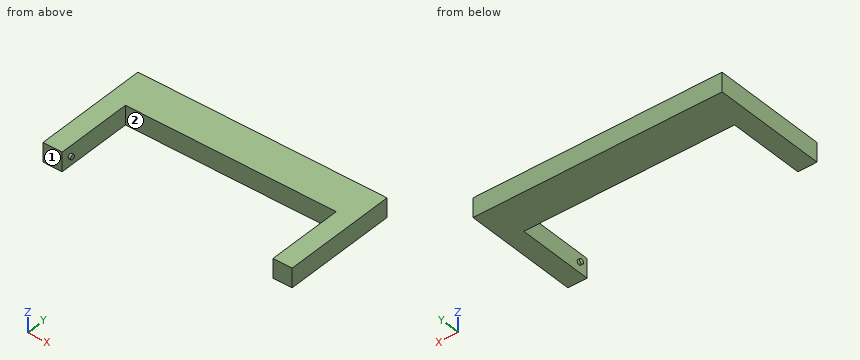
```python
from build123d import *

# Parameters (mm, degrees)
F0_W     = 279.4
F0_H     = 50.8
F1_DEPTH = 25.4
F2_R     = 3.175
F3_DEPTH = 3.175


with BuildPart() as f1:
    # F0 (on Top) → F1 (new body)
    with BuildSketch(Plane.XY):
        with Locations((0, 52.668456)):
            Rectangle(F0_W, F0_H)
        Polygon((-139.7, -74.331544), (-139.7, 27.268456), (-139.7, 78.068456), (-165.1, 78.068456), (-165.1, -74.331544), align=None)
        Polygon((139.7, 78.068456), (139.7, 27.268456), (139.7, -74.331544), (165.1, -74.331544), (165.1, 78.068456), align=None)
    extrude(amount=F1_DEPTH)

    # F2 (on face) → F3 (join)
    with BuildSketch(Plane.YZ.offset(-139.7)):
        with Locations((-61.631544, 12.7)):
            Circle(F2_R)
    extrude(amount=F3_DEPTH)

    # F4: F1 across plane


with BuildPart() as f1_1:
    add(f1.part)
    add(f1.part.mirror(Plane.YZ))


solid = f1_1.part
```
Could you check a few things on this model? Use its own coordinates, in mm. Face numbers are marked on the shaded views. Coordinates: 2 decimals unless noted, no trailing zeros. Loops run counter-clockwise (first coordinate to the right, second up) from the corner with the lowest first, then second, coordinate; pieces in that order, holes last.
1) Please list where these lines run through material, in increasing order: line 1 along X through (y, z) = (-2.5, 13.75); line 2 along Y through (x, z) = (-116, 16).
Reported:
line 1: x = -165.1 to -139.7, 139.7 to 165.1
line 2: y = 27.27 to 78.07
2) Thinking about a two-plate mould opening in X: for the marked faces 1 and 2, which applies, released by +X, released by -X, zero draft, split by the parting line, or undercut?
Reported:
face 1: zero draft
face 2: undercut
3) Imagine slicing it at A-A (y = -43). List the corners of the cut face in (x, z) for me, and give its area (3 significant figures).
Reported:
outline: (-165.1, 0) - (-139.7, 0) - (-139.7, 25.4) - (-165.1, 25.4) - close; (139.7, 0) - (165.1, 0) - (165.1, 25.4) - (139.7, 25.4) - close
area: 1,290 mm2
4) Imagine slicing it at B-B (z = 12.7). List the corners of the cut face in (x, y) for me (3 decimals).
Reported:
outline: (-165.1, -74.332) - (-139.7, -74.332) - (-139.7, -64.807) - (-136.525, -64.807) - (-136.525, -58.457) - (-139.7, -58.457) - (-139.7, 27.268) - (139.7, 27.268) - (139.7, -58.457) - (136.525, -58.457) - (136.525, -64.807) - (139.7, -64.807) - (139.7, -74.332) - (165.1, -74.332) - (165.1, 78.068) - (-165.1, 78.068) - close
5) Imagine slicing it at C-C (x = -38.5). List the corners of the cut face in (y, z) for me.
Reported:
outline: (27.27, 0) - (78.07, 0) - (78.07, 25.4) - (27.27, 25.4) - close
6) Will these pins go through, and if not, where does the flat tip stop? pin 1 Ø10 at (x, y) = (23.5, 50) entering from -Z; pin 2 Ø5 at (x, z) = (90, 8) entering from -Y.
Reported:
pin 1: stops at z = 0
pin 2: stops at y = 27.27
